Here's how the part is built. I have some questions about the finished solid (model axes, mm). Give positions to 0.01 mm unless a question says otherwise; leave off trailing zeros. Order: outer loops, then holes, each group sorted by start corner. A loop starts at its lowest first (then second) coordinate and runs counter-clockwise, first axis right, second up. Notation, with made-up numbers: M 60,74.5 L 96,74.5 A14 cw 96,83.5 Z; hole C 48,48.5 d11. An arc over 180 degrees is marked long. Use one line per item in the form item = value.
from build123d import *

# Parameters (mm, degrees)
F0_R     = 30
F1_DEPTH = 6.35
F3_D     = 10
F5_D     = 4.5
F6_D     = 2.7051
F7_D     = 2.7051
F9_D     = 6.35
F10_D    = 2.7051


with BuildPart() as f1:
    # F0 (on Top) → F1 (new body)
    with BuildSketch(Plane.XY):
        Polygon((-180, 60), (-120, 0), (120, 0), (180, 60), (180, 220), (120, 280), (-120, 280), (-180, 220), align=None)
        with Locations((0, 140)):
            Circle(F0_R, mode=Mode.SUBTRACT)
    extrude(amount=F1_DEPTH)

    # F3 (through all)
    with Locations(Plane.XY.offset(6.35)):
        with Locations((-123.65, 140), (123.65, 140)):
            Hole(F3_D / 2)

    # F5 (through all)
    with Locations(Plane.XY.offset(6.35)):
        with Locations((-121.2489651369, 251.2489651369), (-151.2489651369, 221.2489651369), (-151.2489651369, 58.7510348631), (-121.2489651369, 28.7510348631), (121.2489651369, 28.7510348631), (151.2489651369, 58.7510348631), (151.2489651369, 221.2489651369), (121.2489651369, 251.2489651369)):
            Hole(F5_D / 2)

    # F6 (through all)
    with Locations(Plane.XY.offset(6.35)):
        with Locations((-150, 235.8578643763), (-135.8578643763, 250)):
            Hole(F6_D / 2)

    # F7 (through all)
    with Locations(Plane.XY.offset(6.35)):
        with Locations((-150, 44.1421356237), (-135.8578643763, 30), (135.8578643763, 250), (150, 235.8578643763), (135.8578643763, 30), (150, 44.1421356237)):
            Hole(F7_D / 2)

    # F9 (through all)
    with Locations(Plane.XY.offset(6.35)):
        with Locations((0, 208.14583), (59.016019942, 174.072915), (-59.016019942, 174.072915), (-59.016019942, 105.927085), (0, 71.85417), (59.016019942, 105.927085)):
            Hole(F9_D / 2)

    # F10 (through all)
    with Locations(Plane.XY.offset(6.35)):
        with Locations((147.7549359697, 247.7549359697), (147.7549359697, 32.2450640303), (-147.7549359697, 32.2450640303), (-147.7549359697, 247.7549359697)):
            Hole(F10_D / 2)


solid = f1.part
Q1. I need wall thicknesses on L1, parallel to Y at x = 150, z = 4.25; L2, parallel to Y at x = 122.5, z = 5; L3, parallel to Y at x = 148.5, z = 5.75. Which ranges of each line are inside material? Lowest first, please.
Found:
L1 = 30 to 42.79, 45.49 to 56.88, 60.62 to 219.38, 223.12 to 234.51, 237.21 to 250
L2 = 2.5 to 26.88, 30.62 to 135.13, 144.87 to 249.38, 253.12 to 277.5
L3 = 28.5 to 31.12, 33.37 to 246.63, 248.88 to 251.5
Q2. I want a section at C-C on z = 5. State how many separate pieces and enclosed holes the cut face has, then the cut area to 3 significant figures.
Found:
separate_pieces = 1
enclosed_holes = 29
area = 90,200 mm²
Q3. Thinking about a two-plate mould opening in Y: for faces 1 (the face through (-150, 250, 3)), 2 (the face through (-6.503, 110.713, 3.131)), 3 (the face through (-3, 173, 6.35)), which applies, +Y half, -Y half, draft (parallel to the pull), parting line (faces both ways), or undercut?
Found:
face_1 = +Y half
face_2 = undercut
face_3 = draft
Q4. I want a section at A-A on y = 140. Write out the boundary of the cut face in (x, z), then the cut area to 3 significant figures.
Found:
outline = M -180,0 L -128.65,0 L -128.65,6.35 L -180,6.35 Z; M -118.65,0 L -30,0 L -30,6.35 L -118.65,6.35 Z; M 30,0 L 118.65,0 L 118.65,6.35 L 30,6.35 Z; M 128.65,0 L 180,0 L 180,6.35 L 128.65,6.35 Z
area = 1,780 mm²
Q5. I'm going to push a flat-ended pin straight in: pin 1 Ø2.5 at (x, y) = (147.75, 247.75) entering from -Z. Where does the tip first touch, or does it pass through?
Found:
pin_1 = through
Q6. I want a section at B-B on y = 261. Write out the boundary of the cut face in (x, z), then the cut area to 3 significant figures.
Found:
outline = M -139,0 L 139,0 L 139,6.35 L -139,6.35 Z
area = 1,770 mm²
